```python
from build123d import *

# Parameters (mm, degrees)
ESQUISSE1_W                   = 145
ESQUISSE1_H                   = 127
BOSS_EXTRU_1_DEPTH            = 1.6
DIAM_TRE_DU_PER_AGE_3_0_3_1_D = 3
ENL_V_MAT_EXTRU_1_REACH       = 98.39
ESQUISSE4_R                   = 1.6


with BuildPart() as part:
    # Esquisse1 → Boss.-Extru.1 (new body)
    with BuildSketch(Plane.XY):
        Rectangle(ESQUISSE1_W, ESQUISSE1_H)
    extrude(amount=BOSS_EXTRU_1_DEPTH)

    # Diamètre du perçage Ø3.0 (3)1 (through all)
    with Locations(Plane(origin=(0, 0, 0), x_dir=(-1, 0, 0), z_dir=(0, 0, -1))):
        with Locations((-68.58, 61.04999644), (-38.1, 61.04999644), (-7.62, 61.04999644), (22.86, 61.04999644), (53.34, 61.04999644), (68.58, 61.04999644), (-68.58, -61.05000356), (-53.34, -61.05000356), (-38.1, -61.05000356), (-22.86, -61.05000356), (-7.62, -61.05000356), (7.62, -61.05000356), (22.86, -61.05000356), (38.1, -61.05000356), (53.34, -61.05000356), (68.58, -61.05000356), (38.1, 61.04999644), (7.62, 61.04999644), (-22.86, 61.04999644), (-53.34, 61.04999644)):
            Hole(DIAM_TRE_DU_PER_AGE_3_0_3_1_D / 2)

    # Esquisse4 → Enlèv. mat.-Extru.1 (cut, up to next)
    with BuildSketch(Plane.XY.offset(1.6), mode=Mode.PRIVATE) as enl_v_mat_extru_1_sk1:
        with Locations((67.8, -22.2)):
            Circle(ESQUISSE4_R)
    enl_v_mat_extru_1_tool1 = extrude(enl_v_mat_extru_1_sk1.sketch, amount=-ENL_V_MAT_EXTRU_1_REACH, mode=Mode.PRIVATE) & part.part
    # Esquisse4 → Enlèv. mat.-Extru.1 (cut, up to next)
    with BuildSketch(Plane.XY.offset(1.6), mode=Mode.PRIVATE) as enl_v_mat_extru_1_sk2:
        with Locations((-5.9, -22.2)):
            Circle(ESQUISSE4_R)
    enl_v_mat_extru_1_tool2 = extrude(enl_v_mat_extru_1_sk2.sketch, amount=-ENL_V_MAT_EXTRU_1_REACH, mode=Mode.PRIVATE) & part.part
    # Esquisse4 → Enlèv. mat.-Extru.1 (cut, up to next)
    with BuildSketch(Plane.XY.offset(1.6), mode=Mode.PRIVATE) as enl_v_mat_extru_1_sk3:
        with Locations((-5.9, 31)):
            Circle(ESQUISSE4_R)
    enl_v_mat_extru_1_tool3 = extrude(enl_v_mat_extru_1_sk3.sketch, amount=-ENL_V_MAT_EXTRU_1_REACH, mode=Mode.PRIVATE) & part.part
    # Esquisse4 → Enlèv. mat.-Extru.1 (cut, up to next)
    with BuildSketch(Plane.XY.offset(1.6), mode=Mode.PRIVATE) as enl_v_mat_extru_1_sk4:
        with Locations((67.8, 31)):
            Circle(ESQUISSE4_R)
    enl_v_mat_extru_1_tool4 = extrude(enl_v_mat_extru_1_sk4.sketch, amount=-ENL_V_MAT_EXTRU_1_REACH, mode=Mode.PRIVATE) & part.part
    add(enl_v_mat_extru_1_tool1.solids().sort_by_distance((67.8, -22.2, 1.6))[0], mode=Mode.SUBTRACT)
    add(enl_v_mat_extru_1_tool2.solids().sort_by_distance((-5.9, -22.2, 1.6))[0], mode=Mode.SUBTRACT)
    add(enl_v_mat_extru_1_tool3.solids().sort_by_distance((-5.9, 31, 1.6))[0], mode=Mode.SUBTRACT)
    add(enl_v_mat_extru_1_tool4.solids().sort_by_distance((67.8, 31, 1.6))[0], mode=Mode.SUBTRACT)


solid = part.part
```
Work out the finished part from the listing and answer in its coordinate system (mm). Round coordinates to 2 decimals unless told otherwise and drop trailing zeros. Order: outer loops, then holes, each group sorted by start corner. A loop starts at its lowest first (then second) coordinate and runs counter-clockwise, first axis right, second up.
Q1. Given pin 1 Ø2.5 at (x, y) = (38.1, -61.05) entering from +Z, flat-ended and moving along its own axis, determine where the tip first touches the part or whether it passes through.
Solution:
pin 1: passes through
Q2. The mould has two halves that part along X. Classify faces 1 (the flat face through (-1, 1, 1.6)), 2 (the cylindrical face through (69.28, -22.81, 0.81)): pulls with the +X half, pulls with the -X half, needs draft (parallel to the pull), parting line crosses it, or undercut.
Solution:
face 1: needs draft
face 2: undercut
Q3. Find the intervals of material crossed by line 1 along Y through (x, z) = (22.86, 0.4); line 2 along Y through (x, z) = (68.58, 1.05); line 3 along Y through (x, z) = (-52.5, 1.25), in increasing order.
Solution:
line 1: y = -63.5 to -62.55, -59.55 to 59.55, 62.55 to 63.5
line 2: y = -63.5 to -62.55, -59.55 to -23.6, -20.8 to 29.6, 32.4 to 59.55, 62.55 to 63.5
line 3: y = -63.5 to -62.29, -59.81 to 59.81, 62.29 to 63.5
Q4. A cutting plane is placed at A-A, the plane y = 31. Determine the outline of the cut face in (x, z).
Solution:
outline: (-72.5, 0) - (-7.5, 0) - (-7.5, 1.6) - (-72.5, 1.6) - close; (-4.3, 0) - (66.2, 0) - (66.2, 1.6) - (-4.3, 1.6) - close; (69.4, 0) - (72.5, 0) - (72.5, 1.6) - (69.4, 1.6) - close
